from build123d import *

# Parameters (mm, degrees)
BOSS_EXTRUDE1_DEPTH  = 5.588
SKETCH2_W            = 38.1
SKETCH2_H            = 114.3
BOSS_EXTRUDE2_DEPTH  = 0.762
CUT_EXTRUDE1_DEPTH   = 109.03221727
HOLE1_D              = 8.3312
HOLE2_D              = 8.3312
HOLE3_D              = 8.3312
M8_CLEARANCE_HOLE1_D = 9.525


with BuildPart() as part:
    # Sketch1 → Boss-Extrude1 (new body)
    with BuildSketch(Plane(origin=(0, 0, -17.198296107), x_dir=(-1, 0, 0), z_dir=(0, 0, -1))):
        Polygon((-47.86260239, 85.004743533), (-47.86260239, 46.904743533), (28.33739761, -29.295256467), (66.43739761, -29.295256467), (66.43739761, 85.004743533), align=None)
    extrude(amount=-BOSS_EXTRUDE1_DEPTH)

    # Sketch2 → Boss-Extrude2 (add)
    with BuildSketch(Plane.XY.offset(-11.610296107)):
        with Locations((-47.38739761, 27.854743533)):
            Rectangle(SKETCH2_W, SKETCH2_H)
    extrude(amount=BOSS_EXTRUDE2_DEPTH)

    # Sketch3 → Cut-Extrude1 (cut, through all)
    with BuildSketch(Plane.XY.offset(-11.610296107)):
        with BuildLine():
            ThreePointArc((-9.28739761, 23.689143533), (20.598894761, 36.068451162), (32.97820239, 65.954743533))
            ThreePointArc((32.97820239, 65.954743533), (28.81260239, 70.120343533), (24.64700239, 65.954743533))
            ThreePointArc((24.64700239, 65.954743533), (14.707846746, 41.959499178), (-9.28739761, 32.020343533))
            ThreePointArc((-9.28739761, 32.020343533), (-13.45299761, 27.854743533), (-9.28739761, 23.689143533))
        make_face()
    extrude(amount=-CUT_EXTRUDE1_DEPTH, mode=Mode.SUBTRACT)

    # Hole1 (through all)
    with Locations(Plane.XY.offset(-10.848296107)):
        with Locations((-47.38739761, -10.245256467)):
            Hole(HOLE1_D / 2)

    # Hole2 (through all)
    with Locations(Plane.XY.offset(-10.848296107)):
        with Locations((-47.38739761, 65.954743533)):
            Hole(HOLE2_D / 2)

    # Hole3 (through all)
    with Locations(Plane.XY.offset(-10.848296107)):
        with Locations((-47.38739761, 27.854743533)):
            Hole(HOLE3_D / 2)

    # M8 Clearance Hole1 (through all)
    with Locations(Plane.XY.offset(-11.610296107)):
        with Locations((-9.28739761, 65.954743533)):
            Hole(M8_CLEARANCE_HOLE1_D / 2)


solid = part.part
For this review, take the finished solid that the model builds, in its own axes (mm). A direction names the side the tool comes from. Coordinates: 2 decimals unless noted, no trailing zeros. Order: outer loops, then holes, each group sorted by start corner. A loop starts at its lowest first (then second) coordinate and runs counter-clockwise, first axis right, second up. Notation, with made-up numbers: (75.25, 64) - (97.25, 64) arc R9 ccw to (97.25, 81) - close; hole circle Ø4 at (-33.5, -6.5). An arc over 180 degrees is marked (long way). Answer as CSV lines item,"result". Start each with the question number.
1) Add section B-B (x = -12). State the section outline as (y, z) points.
2) Add section D-D (y = 30). State the section outline as (x, z) points.
3) Machinability: for faces 4 (the cylindrical face through (20.268, 35.742, -14.365)), 5 (the flat face through (-21, 41, -17.198)), which of the approach directions +Z, -Z, +X, -X, +Y, -Y give a long, thin tool a straight path to every point of the face, cutting with its end or side? Answer none if there is none.
4) Insertion check: P1, Ø8, axis at x = 10.5, y = -1, coming from the -Z side. The pin has a flat end and moves straight along its axis. Give the tip position at first contact, or say it passes through.
5) Add section A-A (y = -8.5). State the section outline as (x, z) points.
6) Draft analysis for pull direction X (two halves, no side actions). For faces 1 (the flat face through (47.863, 66, -14)), 2 (the cylindrical face through (-43.226, -10.062, -14.068)), 3 (the flat face through (2, 41, -11.61)), state which applies: +X half, -X half, draft (parallel to the pull), parting line (faces both ways), or undercut.
7) To check wall thickness, follow line 1 along Y through (x, z) = (-7.5, -13.75); line 2 along Z through (x, y) = (-22.5, -12); line 3 along Y through (x, z) = (-4, -12). State the ranges of each line that lie inside material, in increasing order. Write a range as [from, to].
8) Add section C-C (z = -15.25). State the section outline as (x, y) points (1 decimal), then the cut area to 3 significant figures.
Result:
1,outline,"(-12.96, -17.2) - (24.69, -17.2) - (24.69, -11.61) - (-12.96, -11.61) - close; (31.02, -17.2) - (62.04, -17.2) - (62.04, -11.61) - (31.02, -11.61) - close; (69.87, -17.2) - (85, -17.2) - (85, -11.61) - (69.87, -11.61) - close"
2,outline,"(-66.44, -17.2) - (-50.96, -17.2) - (-50.96, -10.85) - (-66.44, -10.85) - close; (-43.82, -17.2) - (-12.86, -17.2) - (-12.86, -11.61) - (-28.34, -11.61) - (-28.34, -10.85) - (-43.82, -10.85) - close; (12.93, -17.2) - (30.96, -17.2) - (30.96, -11.61) - (12.93, -11.61) - close"
3,face 4,"+Z, -Z"
3,face 5,"-Z, +X, -X, +Y, -Y"
4,P1,"through"
5,outline,"(-66.44, -17.2) - (-51.17, -17.2) - (-51.17, -10.85) - (-66.44, -10.85) - close; (-43.61, -17.2) - (-7.54, -17.2) - (-7.54, -11.61) - (-28.34, -11.61) - (-28.34, -10.85) - (-43.61, -10.85) - close"
6,face 1,"+X half"
6,face 2,"undercut"
6,face 3,"draft"
7,line 1,"[-8.46, 23.73], [32.07, 61.54], [70.37, 85]"
7,line 2,"[-17.2, -11.61]"
7,line 3,"[-4.96, 24.02], [32.43, 85]"
8,outline,"(-66.4, -29.3) - (-28.3, -29.3) - (47.9, 46.9) - (47.9, 85) - (-66.4, 85) - close; hole circle Ø8.3 at (-47.4, -10.2); hole circle Ø8.3 at (-47.4, 27.9); hole circle Ø8.3 at (-47.4, 66); hole circle Ø9.5 at (-9.3, 66); hole (-9.3, 23.7) arc R42.3 ccw to (33, 66) arc R4.2 ccw to (24.6, 66) arc R33.9 cw to (-9.3, 32) arc R4.2 ccw to start"
8,area,"9,370 mm^2"
